Autodesk Inventor part; units mm, degrees
ref_plane "YZ Plane" through (0, 0, 0) normal (1, 0, 0) x (0, 1, 0)
ref_plane "XZ Plane" through (0, 0, 0) normal (0, 1, 0) x (-1, 0, 0)
ref_plane "XY Plane" through (0, 0, 0) normal (0, 0, 1) x (1, 0, 0)
sketch "Sketch1" plane through (0, 0, 0) normal (0, 0, 1) x (1, 0, 0)
  circle A0 centre (0, 0) radius 12.3
  arc A1 (-26.8669, -23.9619) -> (26.8669, -23.9619) centre (0, 0) ccw
  line L0 (-26.8669, 13.9698) -> (-26.8669, -23.9619)
  line L1 (26.8669, 13.9698) -> (26.8669, -23.9619)
  arc A2 (26.8669, -23.9619) -> (-26.8669, -23.9619) centre (0, 0) ccw construction
  arc A3 (-26.8669, 13.9698) -> (26.8669, 13.9698) centre (0, 0) ccw construction
  arc A4 (26.8669, 13.9698) -> (-26.8669, 13.9698) centre (0, -28.1986) ccw
  line L2 (0, -28.1986) -> (0, 0) construction
  dimension "d0" = 24.6
  dimension "d1" = 72
  dimension "d13" = 50
extrude "Extrusion1" add sketch "Sketch1" along normal blind 3
sketch "Sketch2" plane through (0, 0, 3) normal (0, 0, 1) x (1, 0, 0)
  circle A0 centre (-16, 0) radius 2.25
  circle A1 centre (16, 0) radius 2.25
  circle A2 centre (0, 16) radius 2.25
  line L0 (0, 0) -> (0, 16) construction
  line L1 (0, 0) -> (16, 0) construction
  line L2 (0, 0) -> (-16, 0) construction
  dimension "d5" = 4.5
  dimension "d6" = 4.5
  dimension "d7" = 4.5
  dimension "d8" = 16
  dimension "d9" = 16
  dimension "d10" = 16
extrude "Extrusion2" cut sketch "Sketch2" against normal blind 3
equation "\"d9\" = d8"
equation "\"d10\" = d8"
properties part number "Gear Protection Piece" material "Aluminum 6061"
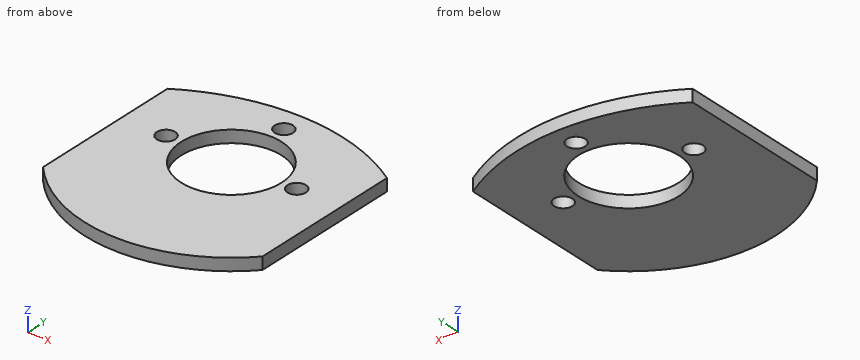
Can you work these out from the model? Positions are in its coordinate system, mm. Round coordinates to 2 decimals unless told otherwise and drop trailing zeros. Write each loop counter-clockwise with the first axis right and the second up, starting at its lowest first coordinate (ties: lowest second). Pieces come first, ordered by that corner, then holes. Notation, with made-up numbers: M 18,-17.75 L 72,-17.75 A15 ccw 72,3.25 Z; hole C 45.5,65 d9. An arc over 180 degrees is marked long. Use a Markdown table: item, result.
Item 1: I want a section at B-B (y = 0). List the corners of the cut face in (x, z) for me, and give its area (3 significant figures).
Found:
| item | result |
|---|---|
| outline | M -26.87,0 L -18.25,0 L -18.25,3 L -26.87,3 Z; M -13.75,0 L -12.3,0 L -12.3,3 L -13.75,3 Z; M 12.3,0 L 13.75,0 L 13.75,3 L 12.3,3 Z; M 18.25,0 L 26.87,0 L 26.87,3 L 18.25,3 Z |
| area | 60.4 mm2 |
Item 2: I want a section at D-D (x = -16). List the corners of the cut face in (y, z) for me, and give its area (3 significant figures).
Found:
| item | result |
|---|---|
| outline | M -32.25,0 L -2.25,0 L -2.25,3 L -32.25,3 Z; M 2.25,0 L 19.17,0 L 19.17,3 L 2.25,3 Z |
| area | 141 mm2 |
Item 3: If I drill on line 1 along Y through (x, z) = (-6.5, 1.15); line 2 along Y through (x, z) = (-10, 0.55); line 3 along X through (y, z) = (5, 0.9), over which ranges is the centre line in solid material (lowest first)? Write a range as [from, to].
Found:
| item | result |
|---|---|
| line 1 | y = [-35.41, -10.44], [10.44, 21.38] |
| line 2 | y = [-34.58, -7.16], [7.16, 20.79] |
| line 3 | x = [-26.87, -11.24], [11.24, 26.87] |
Item 4: I want a section at C-C (z = 1.35). List the corners of the cut face in (x, y) for me, and give its area (3 significant figures).
Found:
| item | result |
|---|---|
| outline | M -26.87,-23.96 A36 ccw 26.87,-23.96 L 26.87,13.97 A50 ccw -26.87,13.97 Z; hole C -16,0 d4.5; hole C 0,0 d24.6; hole C 0,16 d4.5; hole C 16,0 d4.5 |
| area | 2,250 mm2 |
Item 5: I want a section at A-A (x = 0). List the corners of the cut face in (y, z) for me.
Found:
| item | result |
|---|---|
| outline | M -36,0 L -12.3,0 L -12.3,3 L -36,3 Z; M 12.3,0 L 13.75,0 L 13.75,3 L 12.3,3 Z; M 18.25,0 L 21.8,0 L 21.8,3 L 18.25,3 Z |
